from build123d import *

# Parameters (mm, degrees)
SKETCH1_R               = 130
BOSS_EXTRUDE1_DEPTH     = 240
SKETCH2_R               = 105
CUT_EXTRUDE1_DEPTH      = 170
CUT_EXTRUDE2_DEPTH      = 303.324329157
CUT_EXTRUDE2_DEPTH_BACK = 303.324329157
SKETCH3_R               = 12.5
SKETCH3_R_2             = 32.5


with BuildPart() as part:
    # Sketch1 → Boss-Extrude1 (new body)
    with BuildSketch(Plane(origin=(0, 0, 0), x_dir=(1, 0, 0), z_dir=(0, 1, 0))):
        with Locations(Location((0, 0, 0), (0, 0, 270))):
            Circle(SKETCH1_R)
    extrude(amount=BOSS_EXTRUDE1_DEPTH)

    # Sketch2 → Cut-Extrude1 (cut)
    with BuildSketch(Plane(origin=(0, 240, 0), x_dir=(1, 0, 0), z_dir=(0, 1, 0))):
        with Locations(Location((0, 0, 0), (0, 0, 270))):
            Circle(SKETCH2_R)
    extrude(amount=-CUT_EXTRUDE1_DEPTH, mode=Mode.SUBTRACT)

    # Sketch3 → Cut-Extrude2 (cut, two sides: drawn at the far end of the back side and taken through both)
    with BuildSketch(Plane.XZ.offset(-CUT_EXTRUDE2_DEPTH_BACK)):
        with Locations(Location((-90, 0, 0), (0, 0, 90))):
            Circle(SKETCH3_R)
        with Locations(Location((90, 0, 0), (0, 0, 90))):
            Circle(SKETCH3_R)
        with Locations(Location((0, 0, 0), (0, 0, 90))):
            Circle(SKETCH3_R_2)
    extrude(amount=CUT_EXTRUDE2_DEPTH + CUT_EXTRUDE2_DEPTH_BACK, mode=Mode.SUBTRACT)


solid = part.part
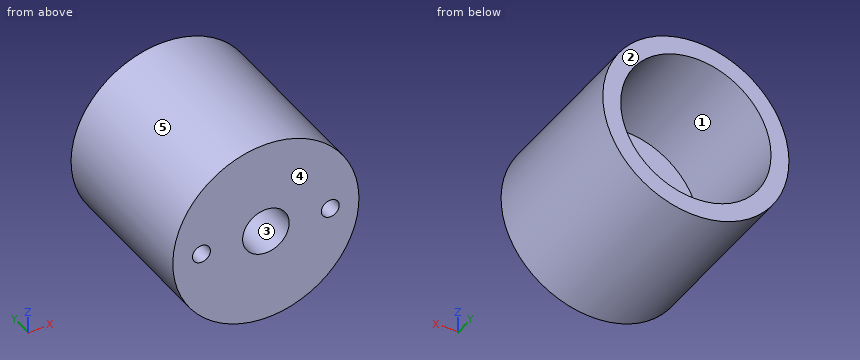
Input: part model. Units: mm. Frame: model coordinates. Face numbers are marked on the shaded views. A direction names the side the tool comes from. Give positions to 0.01 mm unless a question says otherwise; leave off trailing zeros. Write each loop counter-clockwise with the first axis right and the second up, starting at its lowest first coordinate (ties: lowest second). Pieces come first, ordered by that corner, then holes. Notation, with made-up numbers: (-28.75, -38) -> (23.25, -38) arc R12 ccw to (23.25, -16) -> close; hole circle Ø9 at (2.25, 58.5). An arc over 180 degrees is marked (long way). Use one line per item in the form item = value. Start each with the question number.
1) Section query D-D on x = 68. Return the cut outline in (y, z).
2) Set-up query: the marked faces 1 and 2. Return all of +Z, -Z, +X, -X, +Y, -Y with unobstructed straight access to the full face (end or side cutting, diameter ignored); none if empty.
3) Section query B-B on z = 0. Return the cut outline in (x, y).
4) Section query A-A on x = 0. Return the cut outline in (y, z), then the cut area to 4 significant figures.
5) Section query C-C on y = 168. Return the cut outline in (x, z), then the cut area to 3 significant figures.
6) Ray query, probe 1 along X at (y, z) = (23.5, 0); probe 2 along X at (y, z) = (151.5, 0); probe 3 along Z at (x, y) = (3, 140.5). Return the intervals inside material, ascending. Write a range as from..to.
7) Draft query along Z for the marked faces 3, 4 and 5. Return one class per face: pulls with the +Z half, pulls with the -Z half, needs draft (parallel to the pull), parting line crosses it, or undercut.
8) Pin query (flat end, axial travel): pin 1 (3 mm diameter, centred on x = 23, z = 78.5, fed in from +Y); pin 2 (12 mm diameter, centred on x = -92, y = 61.5, fed in from -Z); pin 3 (5 mm diameter, centred on y = 52, z = 15.5, fed in from +X). Return the tip coordinate at first contact, or that it passes through.
Outcome:
q1.outline = (0, -110.8) -> (240, -110.8) -> (240, -80.01) -> (70, -80.01) -> (70, 80.01) -> (240, 80.01) -> (240, 110.8) -> (0, 110.8) -> close
q2.face_1 = +Y
q2.face_2 = +Z, -Z, +X, -X, +Y
q3.outline = (-130, 0) -> (-102.5, 0) -> (-102.5, 70) -> (-105, 70) -> (-105, 240) -> (-130, 240) -> close; (-77.5, 0) -> (-32.5, 0) -> (-32.5, 70) -> (-77.5, 70) -> close; (32.5, 0) -> (77.5, 0) -> (77.5, 70) -> (32.5, 70) -> close; (102.5, 0) -> (130, 0) -> (130, 240) -> (105, 240) -> (105, 70) -> (102.5, 70) -> close
q4.outline = (0, -130) -> (240, -130) -> (240, -105) -> (70, -105) -> (70, -32.5) -> (0, -32.5) -> close; (0, 32.5) -> (70, 32.5) -> (70, 105) -> (240, 105) -> (240, 130) -> (0, 130) -> close
q4.area = 22,150 mm^2
q5.outline = circle Ø260 at (0, 0); hole circle Ø210 at (0, 0)
q5.area = 18,500 mm^2
q6.probe_1 = -130..-102.5, -77.5..-32.5, 32.5..77.5, 102.5..130
q6.probe_2 = -130..-105, 105..130
q6.probe_3 = -129.97..-104.96, 104.96..129.97
q7.face_3 = undercut
q7.face_4 = needs draft
q7.face_5 = parting line crosses it
q8.pin_1 = 70
q8.pin_2 = -97.49
q8.pin_3 = 129.35
